from build123d import *

# Parameters (mm, degrees)
CYLINDER003_R               = 29.7
CYLINDER003_DEPTH           = 10
CYLINDER002_R               = 35
CYLINDER002_DEPTH           = 10
CYLINDER001_W               = 22
CYLINDER001_H               = 10
CYLINDER001_ANGLE           = 18
CYLINDER001_PLACEMENT_ANGLE = -9
ARRAY_COUNT                 = 24
CYLINDER_R                  = 29.7
CYLINDER_DEPTH              = 10


with BuildPart() as obj1:
    # Cylinder003 → Cylinder003 (new body)
    with BuildSketch(Plane.XY):
        Circle(CYLINDER003_R)
    extrude(amount=CYLINDER003_DEPTH)


with BuildPart() as obj2:
    # Cylinder002 → Cylinder002 (new body)
    with BuildSketch(Plane.XY):
        Circle(CYLINDER002_R)
    extrude(amount=CYLINDER002_DEPTH)

    # Cut001: cut obj1
    add(obj1.part, mode=Mode.SUBTRACT)


with BuildPart() as array:
    # Cylinder001 → Cylinder001 (revolve)
    with BuildSketch(Plane.XZ):
        with Locations((11, 5)):
            Rectangle(CYLINDER001_W, CYLINDER001_H)
    revolve(axis=Axis((0, 0, 0), (0, 0, 1)), revolution_arc=CYLINDER001_ANGLE)


with BuildPart() as array_1:
    # Cylinder001 placement: moved
    add(array.part.moved(Location((8, 0, 0))).rotate(Axis((8, 0, 0), (0, 0, 1)), CYLINDER001_PLACEMENT_ANGLE))

    # Array: Array ×24 about axis
    array_axis = Axis((0, 0, 0), (0, 0, 1))


with BuildPart() as array_2:
    add(array_1.part)
    for i in range(1, ARRAY_COUNT):
        add(array_1.part.rotate(array_axis, i * 360 / ARRAY_COUNT))


with BuildPart() as rueda_con_radios:
    # Cylinder → Cylinder (new body)
    with BuildSketch(Plane.XY):
        Circle(CYLINDER_R)
    extrude(amount=CYLINDER_DEPTH)

    # Cut: cut Array
    add(array_2.part, mode=Mode.SUBTRACT)

    # Fusion: union obj2
    add(obj2.part)


solid = rueda_con_radios.part
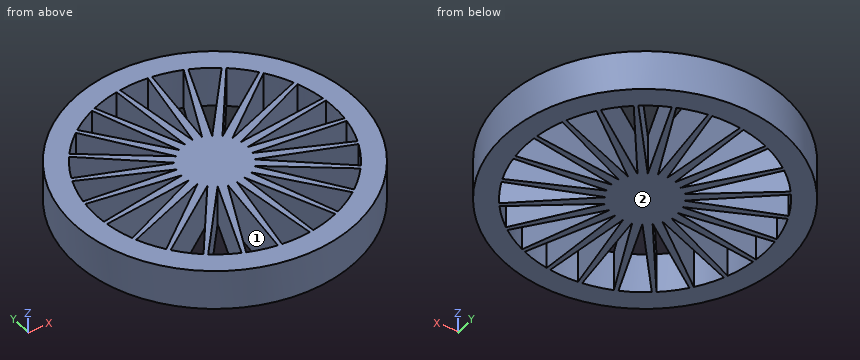
Input: part model. Units: mm. Frame: model coordinates. Face numbers are marked on the shaded views. Coordinates: 2 decimals unless noted, no trailing zeros.
1. Draft query along X for the marked faces 1 and 2. Return one class per face: +X half, -X half, draft (parallel to the pull), parting line (faces both ways), or undercut.
Checked values:
face 1: undercut
face 2: draft
2. Contact query for flat-ended pins moving along their axis: P1, Ø5, axis at x = -2.5, z = 8.5, coming from the -Y side; P2, Ø2, axis at x = 6.5, z = 3, coming from the +Y side; P3, Ø1.5, axis at x = 25.5, z = 5, coming from the -Y side. Output: stop coordinate, or through.
Checked values:
P1: stops at y = -35
P2: stops at y = 34.57
P3: stops at y = -24.75
3. Cut plane A-A, the plane z = 7.75. Count the separate pieces of the cut face and the enclosed holes in it, plus the area to 3 significant figures.
Checked values:
separate pieces: 1
enclosed holes: 24
area: 2,070 mm2
4. Ray query, line 1 along X through (y, z) = (-24, 1.5); line 2 along X through (y, z) = (-27, 9.5). Return the intervals inside material, ascending.
Checked values:
line 1: x = -25.48 to -17.5, -10.55 to -9.32, -3.78 to -2.53, 2.53 to 3.78, 9.32 to 10.55, 17.5 to 25.48
line 2: x = -22.27 to -12.37, -11.7 to -10.65, -4.1 to -3.01, 3.01 to 4.1, 10.65 to 11.7, 12.37 to 22.27
